Here's how the part is built. I have some questions about the finished solid (model axes, mm). A direction names the side the tool comes from. Round coordinates to 2 decimals unless told otherwise and drop trailing zeros. Order: outer loops, then holes, each group sorted by start corner. A loop starts at its lowest first (then second) coordinate and runs counter-clockwise, first axis right, second up. Notation, with made-up numbers: (33, 63.25) - (64, 63.25) arc R34 ccw to (64, 101.25) - close; hole circle Ø10 at (-16, 8). An arc over 180 degrees is marked (long way). Answer as a JSON object with one key per item and string values.
```python
from build123d import *

# Parameters (mm, degrees)
SKETCH_1_R          = 24.75
SKETCH_1_R_2        = 17.5
EXTRUDE_1_DEPTH     = 3.5
SKETCH_2_R          = 27
SKETCH_2_R_2        = 17.5
EXTRUDE_2_DEPTH     = 7
SKETCH_3_R          = 2
CUT_EXTRUDE_1_DEPTH = 15
EXTRUDE_3_DEPTH     = 5


with BuildPart() as part:
    # 草图1 → 凸台-拉伸1 (new, symmetric)
    with BuildSketch(Plane.XY):
        Circle(SKETCH_1_R)
        Circle(SKETCH_1_R_2, mode=Mode.SUBTRACT)
    extrude(amount=EXTRUDE_1_DEPTH, both=True)

    # 草图2 → 凸台-拉伸2 (add)
    with BuildSketch(Plane.XY.offset(3.5)):
        Circle(SKETCH_2_R)
        Circle(SKETCH_2_R_2, mode=Mode.SUBTRACT)
    extrude(amount=EXTRUDE_2_DEPTH)

    # 草图3 → 切除-拉伸1 (cut)
    with BuildSketch(Plane(origin=(0, 0, -3.5), x_dir=(-1, 0, 0), z_dir=(0, 0, -1))):
        with Locations((14.849242405, 14.849242405)):
            Circle(SKETCH_3_R)
        with Locations((14.849242405, -14.849242405)):
            Circle(SKETCH_3_R)
        with Locations((-14.849242405, -14.849242405)):
            Circle(SKETCH_3_R)
        with Locations((-14.849242405, 14.849242405)):
            Circle(SKETCH_3_R)
    extrude(amount=-CUT_EXTRUDE_1_DEPTH, mode=Mode.SUBTRACT)

    # 草图4 → 凸台-拉伸3 (add)
    with BuildSketch(Plane(origin=(0, 0, 3.5), x_dir=(-1, 0, 0), z_dir=(0, 0, -1))):
        with BuildLine():
            ThreePointArc((27, 0), (1.450134249, 26.961029481), (-26.844230419, 2.896082389))
            Line((-26.844230419, 2.896082389), (-24.579975728, 2.896082389))
            ThreePointArc((-24.579975728, 2.896082389), (1.45053451, 24.707457369), (24.75, 0))
            ThreePointArc((24.75, 0), (1.45053451, -24.707457369), (-24.579975728, -2.896082389))
            Line((-24.579975728, -2.896082389), (-26.844230419, -2.896082389))
            ThreePointArc((-26.844230419, -2.896082389), (1.450134249, -26.961029481), (27, 0))
        make_face()
        with BuildLine():
            Line((-24.579975728, 2.896082389), (-26.844230419, 2.896082389))
            ThreePointArc((-26.844230419, 2.896082389), (-27, 0), (-26.844230419, -2.896082389))
            Line((-26.844230419, -2.896082389), (-24.579975728, -2.896082389))
            ThreePointArc((-24.579975728, -2.896082389), (-24.75, 0), (-24.579975728, 2.896082389))
        make_face()
        with BuildLine():
            Line((-26.844230419, 2.896082389), (-34.879975728, 2.896082389))
            ThreePointArc((-34.879975728, 2.896082389), (-35, 0), (-34.879975728, -2.896082389))
            Line((-34.879975728, -2.896082389), (-26.844230419, -2.896082389))
            ThreePointArc((-26.844230419, -2.896082389), (-27, 0), (-26.844230419, 2.896082389))
        make_face()
    extrude(amount=-EXTRUDE_3_DEPTH)


solid = part.part
```
1. Imagine slicing it at D-D (y = 23.5). List the corners of the cut face in (x, z) for me.
Responses:
{"outline": "(-13.29, 3.5) - (-7.77, 3.5) - (-7.77, -3.5) - (7.77, -3.5) - (7.77, 3.5) - (13.29, 3.5) - (13.29, 10.5) - (-13.29, 10.5) - close"}
2. Thinking about a two-plate mould opening in Y: for faces 1 (the face through (31, -2.896, 6)), 2 (the face through (16.847, 14.937, 3.402)), 3 (the face through (31, 2.896, 6)), which applies, pulls with the +Y half, pulls with the -Y half, needs draft (parallel to the pull), parting line crosses it, or undercut?
Responses:
{"face 1": "pulls with the -Y half", "face 2": "undercut", "face 3": "pulls with the +Y half"}
3. Imagine slicing it at B-B (z = 7.75). List the corners of the cut face in (x, y) for me.
Responses:
{"outline": "(26.84, -2.9) - (34.88, -2.9) arc R35 ccw to (34.88, 2.9) - (26.84, 2.9) arc R27 ccw (long way) to start; hole circle Ø35 at (0, 0); hole circle Ø4 at (-14.85, -14.85); hole circle Ø4 at (-14.85, 14.85); hole circle Ø4 at (14.85, -14.85); hole circle Ø4 at (14.85, 14.85)"}
4. For P1, Ø4, axis at y = 14, z = 3, coming from the +X side; P2, Ø3, axis at x = 12.5, z = 2.5, coming from the -Y side; P3, Ø1.5, axis at x = 31, z = 5.5, coming from the -Y side, each with a flat end and sliding along its axis, tell me the tip position at first contact or that it passes through.
Responses:
{"P1": "x = 24.16", "P2": "y = -24.48", "P3": "y = -2.9"}
5. For faces 4 (the face through (-3.22, 24.54, 0.05)), 5 (the face through (18, 0, 10.5)), which set-ups out of +Z, -Z, +X, -X, +Y, -Y let a thin tool reach every point of the face, with its end or its side?
Responses:
{"face 4": "-Z", "face 5": "+Z, +X, -X, +Y, -Y"}
6. Imagine slicing it at A-A (x = 0). List the corners of the cut face in (y, z) for me, plus the area to 4 significant figures.
Responses:
{"outline": "(-27, 3.5) - (-24.75, 3.5) - (-24.75, -3.5) - (-17.5, -3.5) - (-17.5, 10.5) - (-27, 10.5) - close; (17.5, -3.5) - (24.75, -3.5) - (24.75, 3.5) - (27, 3.5) - (27, 10.5) - (17.5, 10.5) - close", "area": "234.5 mm2"}
7. Imagine slicing it at C-C (y = -2). List the corners of the cut face in (x, z) for me, plus the area to 3 significant figures.
Responses:
{"outline": "(-26.93, 3.5) - (-24.67, 3.5) - (-24.67, -3.5) - (-17.39, -3.5) - (-17.39, 10.5) - (-26.93, 10.5) - close; (17.39, -3.5) - (24.67, -3.5) - (24.67, 3.5) - (34.94, 3.5) - (34.94, 8.5) - (26.93, 8.5) - (26.93, 10.5) - (17.39, 10.5) - close", "area": "276 mm2"}
8. If I drill on L1, parallel to Y at x = 15, z = 3; L2, parallel to Y at x = 15, z = 5.5; L3, parallel to Y at x = 0, z = 6.5, over which ranges is the centre line in solid material (lowest first)? Write a range as [from, to].
Responses:
{"L1": "[-19.69, -16.84], [-12.85, -9.01], [9.01, 12.85], [16.84, 19.69]", "L2": "[-22.45, -16.84], [-12.85, -9.01], [9.01, 12.85], [16.84, 22.45]", "L3": "[-27, -17.5], [17.5, 27]"}
